```python
from build123d import *

# Parameters (mm, degrees)
SKETCH1_R           = 40
SKETCH1_R_2         = 1.5
BOSS_EXTRUDE1_DEPTH = 3
SKETCH2_R           = 1.5
CUT_EXTRUDE1_DEPTH  = 3


with BuildPart() as part:
    # Sketch1 → Boss-Extrude1 (new body)
    with BuildSketch(Plane(origin=(0, 0, 0), x_dir=(1, 0, 0), z_dir=(0, 1, 0))):
        Circle(SKETCH1_R)
        with Locations((0, 35)):
            Circle(SKETCH1_R_2, mode=Mode.SUBTRACT)
        with Locations((35, 0)):
            Circle(SKETCH1_R_2, mode=Mode.SUBTRACT)
        with Locations((0, -35)):
            Circle(SKETCH1_R_2, mode=Mode.SUBTRACT)
        with Locations((-35, 0)):
            Circle(SKETCH1_R_2, mode=Mode.SUBTRACT)
    extrude(amount=BOSS_EXTRUDE1_DEPTH)

    # Sketch2 → Cut-Extrude1 (cut)
    with BuildSketch(Plane(origin=(0, 3, 0), x_dir=(1, 0, 0), z_dir=(0, 1, 0))):
        with Locations((10, 10)):
            Circle(SKETCH2_R)
        with Locations((-10, 10)):
            Circle(SKETCH2_R)
        with Locations((-10, -10)):
            Circle(SKETCH2_R)
        with Locations((10, -10)):
            Circle(SKETCH2_R)
    extrude(amount=-CUT_EXTRUDE1_DEPTH, mode=Mode.SUBTRACT)


solid = part.part
```
The model under review builds one solid part; all positions refer to its coordinate system, in mm. Coordinates: 2 decimals unless noted, no trailing zeros. Write each loop counter-clockwise with the first axis right and the second up, starting at its lowest first coordinate (ties: lowest second). Pieces come first, ordered by that corner, then holes. Notation, with made-up numbers: (-36.5, 2.25) - (-2.5, 2.25) arc R16 ccw to (-2.5, 15.25) - close; hole circle Ø10 at (78, -39). An arc over 180 degrees is marked (long way). Answer in a Markdown table with one row per item. Add a question column.
Q1. To check wall thickness, follow line 1 along Z through (x, y) = (0, 0.8); line 2 along Z through (x, y) = (10, 1.55); line 3 along X through (y, z) = (0.4, -0.5). State the ranges of each line that lie inside material, in increasing order. Write a range as from..to.
Q2. Consider section A-A on y = 1.3. Give the number of separate pieces and of enclosed holes in the cut face, then the cut area to 3 significant figures.
Q3. Draft analysis for pull direction Z (two halves, no side actions). For faces 1 (the face through (-8.67, 1.48, 39.05)), 2 (the face through (-11.2, 1.5, -9.1)), 3 (the face through (-1, 0, -1)), state which applies: +Z half, -Z half, draft (parallel to the pull), parting line (faces both ways), or undercut.
Q4. Consider section B-B on x = -35. Give the boundary of the cut face in (y, z), then the cut area to 3 significant figures.
Q5. Consider section C-C on z = 35. Give the boundary of the cut face in (x, y), then the cut area to 3 significant figures.
Q6. Consider section D-D on x = 10. Give the boundary of the cut face in (y, z).
Answers below:
| question | item | result |
|---|---|---|
| 1 | line 1 | -40..-36.5, -33.5..33.5, 36.5..40 |
| 1 | line 2 | -38.73..-11.5, -8.5..8.5, 11.5..38.73 |
| 1 | line 3 | -40..-36.41, -33.59..33.59, 36.41..40 |
| 2 | separate pieces | 1 |
| 2 | enclosed holes | 8 |
| 2 | area | 4,970 mm² |
| 3 | face 1 | parting line |
| 3 | face 2 | undercut |
| 3 | face 3 | draft |
| 4 | outline | (0, -19.36) - (3, -19.36) - (3, -1.5) - (0, -1.5) - close; (0, 1.5) - (3, 1.5) - (3, 19.36) - (0, 19.36) - close |
| 4 | area | 107 mm² |
| 5 | outline | (-19.36, 0) - (-1.5, 0) - (-1.5, 3) - (-19.36, 3) - close; (1.5, 0) - (19.36, 0) - (19.36, 3) - (1.5, 3) - close |
| 5 | area | 107 mm² |
| 6 | outline | (0, -38.73) - (3, -38.73) - (3, -11.5) - (0, -11.5) - close; (0, -8.5) - (3, -8.5) - (3, 8.5) - (0, 8.5) - close; (0, 11.5) - (3, 11.5) - (3, 38.73) - (0, 38.73) - close |
